Part model, mm, in its own coordinate system. A direction names the side the tool comes from. Round coordinates to 2 decimals unless told otherwise and drop trailing zeros. Loops run counter-clockwise (first coordinate to the right, second up) from the corner with the lowest first, then second, coordinate; pieces in that order, holes last.
from build123d import *

# Parameters (mm, degrees)
F0_R          = 6
F1_DEPTH      = 115
F2_W          = 1
F2_H          = 10
F3_DEPTH      = 6.001
F3_DEPTH_BACK = 6.001
F4_SIZE2      = 1
F4_SIZE       = 1


with BuildPart() as f1:
    # F0 (on Top) → F1 (new body)
    with BuildSketch(Plane.XY):
        Circle(F0_R)
    extrude(amount=-F1_DEPTH)

    # F2 (on Front) → F3 (cut, two sides)
    with BuildSketch(Plane.XZ) as f3_sk:
        with Locations((5.5, -13)):
            Rectangle(F2_W, F2_H)
        with Locations((-5.5, -13)):
            Rectangle(F2_W, F2_H)
    extrude(amount=-F3_DEPTH, mode=Mode.SUBTRACT)
    extrude(f3_sk.sketch, amount=F3_DEPTH_BACK, mode=Mode.SUBTRACT)

    # F4
    f4_edges = [f1.edges().sort_by_distance(p)[0] for p in [
        (-6, 0, 0),
        (-6, 0, -115),
    ]]
    chamfer(f4_edges, length=F4_SIZE, length2=F4_SIZE2)


solid = f1.part
1) Mould opens along Z. For faces 3 (the face through (-6, 0, -57)), 4 (the face through (-5, 0, -13)), 5 (the face through (0, 0, -115)) say: released by +Z, released by -Z, zero draft, split by the parting line, or undercut.
Values:
face 3: zero draft
face 4: undercut
face 5: released by -Z
2) Drop flat-ended pins along their axis: pin 1 Ø4 at (y, z) = (4, -57) entering from -X; pin 2 Ø1.1 at (x, y) = (5.5, -1.5) entering from -Z; pin 3 Ø0.8 at (x, y) = (-5.5, 0.5) entering from -Z. Give the stop position or say it passes through.
Values:
pin 1: stops at x = -5.66
pin 2: stops at z = -114.85
pin 3: stops at z = -114.88
3) Wall check: line 1 along X through (y, z) = (-1.25, -9.5); line 2 along Y through (x, z) = (5, -64). Give the ranges that are in metal, low to high.
Values:
line 1: x = -5 to 5
line 2: y = -3.32 to 3.32
4) Slice it at B-B, the plane z = -37. Give the cut face in (x, y), then the cut area to 3 significant figures.
Values:
outline: circle Ø12 at (0, 0)
area: 113 mm2
5) Slice it at A-A, the plane y = 0. Give the cut face in (x, z).
Values:
outline: (-6, -114) - (-5, -115) - (5, -115) - (6, -114) - (6, -18) - (5, -18) - (5, -8) - (6, -8) - (6, -1) - (5, 0) - (-5, 0) - (-6, -1) - (-6, -8) - (-5, -8) - (-5, -18) - (-6, -18) - close
6) Tool access for faces 1 (the face through (0, 0, 0)), 2 (the face through (5, 0, -13)): list every direction of +Z, -Z, +X, -X, +Y, -Y with a clear straight run to the whole face (end or side of a thin tool).
Values:
face 1: +Z, +X, -X, +Y, -Y
face 2: +X, +Y, -Y
